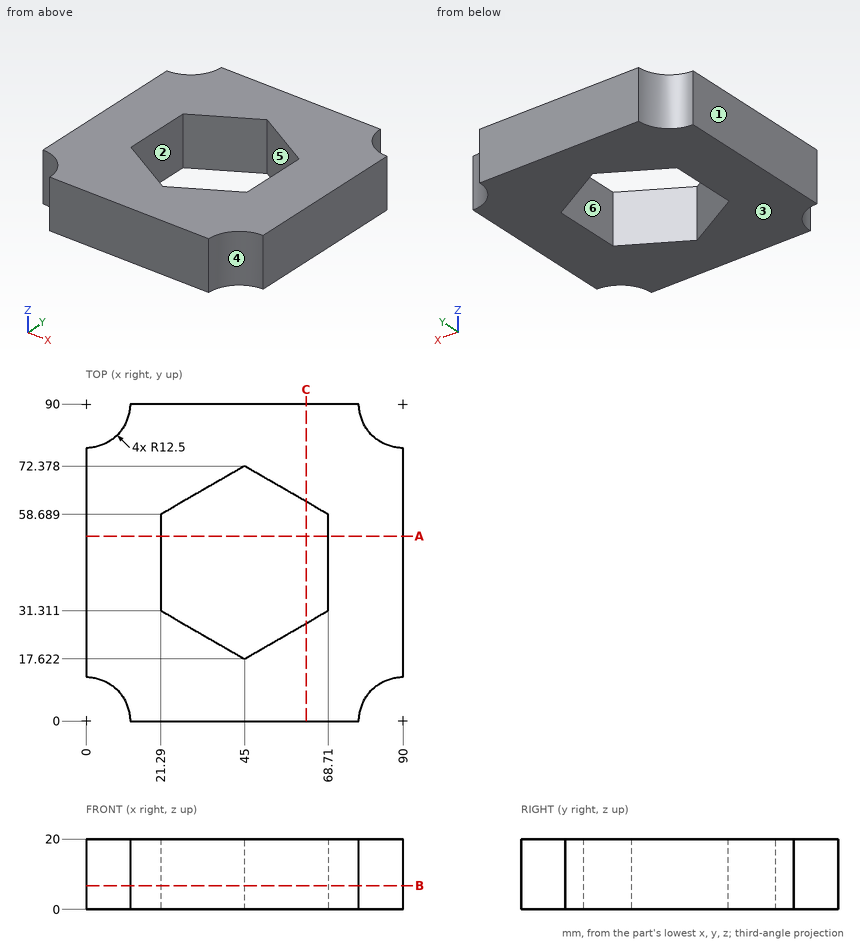
Here's the drawing with two shaded views (mm, measured from the low corner). I have some questions. A direction names the side the tool comes from. Round coordinates to 2 decimals unless told otherwise and drop trailing zeros. Write each loop counter-clockwise with the first axis right and the second up, starting at its lowest first coordinate (ties: lowest second). Pieces come first, ordered by that corner, then holes. Notation, with made-up numbers: M 68,-4.75 L 94,-4.75 A32 cw 94,30.25 Z; hole C -20.75,70.5 d1. An arc over 180 degrees is marked long. Answer in a Markdown table with one row per item. Add a question column.
Q1. If I drill on line 1 (X direction, y = 58.5, z = 5.25); line 2 (Y direction, x = 23, z = 13); line 3 (X direction, y = 29, z = 7.75), over which ranges is the centre line in solid material (lowest first)? Write a range as from..to.
Q2. On a 3-axis mill with a long thin cutter (end or side, diameter ignored), from which of +Z, -Z, +X, -X, +Y, -Y can I reach the whole of each face in a straight line? I mean the marked faces 1 and 2. Say none if no direction works.
Q3. Imagine slicing it at C-C (x = 62.5). Please give me the cut outline in (y, z).
Q4. If we mould it in two halves opening along Y, with no side actions, what happens to the marked faces 3, 4, 5 and 6? For each: +Y half, -Y half, draft (parallel to the pull), parting line (faces both ways), or undercut.
Q5. Imagine slicing it at A-A (y = 52.5). Please give me the cut outline in (x, z).
Q6. Imagine slicing it at B-B (z = 6.75). Please give me the cut outline in (x, y).
Values:
| question | item | result |
|---|---|---|
| 1 | line 1 | 0..21.29, 68.71..90 |
| 1 | line 2 | 0..30.32, 59.68..90 |
| 1 | line 3 | 0..25.29, 64.71..90 |
| 2 | face 1 | +Z, -Z, -X, +Y, -Y |
| 2 | face 2 | +Z, -Z |
| 3 | outline | M 0,0 L 27.73,0 L 27.73,20 L 0,20 Z; M 62.27,0 L 90,0 L 90,20 L 62.27,20 Z |
| 4 | face 3 | draft |
| 4 | face 4 | -Y half |
| 4 | face 5 | undercut |
| 4 | face 6 | undercut |
| 5 | outline | M 0,0 L 21.29,0 L 21.29,20 L 0,20 Z; M 68.71,0 L 90,0 L 90,20 L 68.71,20 Z |
| 6 | outline | M 0,12.5 A12.5 cw 12.5,0 L 77.5,0 A12.5 cw 90,12.5 L 90,77.5 A12.5 cw 77.5,90 L 12.5,90 A12.5 cw 0,77.5 Z; hole M 21.29,31.31 L 45,17.62 L 68.71,31.31 L 68.71,58.69 L 45,72.38 L 21.29,58.69 Z |
